Autodesk Inventor part; units mm, degrees
ref_plane "YZ Plane" through (0, 0, 0) normal (1, 0, 0) x (0, 1, 0)
ref_plane "XZ Plane" through (0, 0, 0) normal (0, 1, 0) x (-1, 0, 0)
ref_plane "XY Plane" through (0, 0, 0) normal (0, 0, 1) x (1, 0, 0)
sketch "Sketch1" plane through (0, 0, 0) normal (0, 0, 1) x (1, 0, 0)
  circle A0 centre (0, 0) radius 3.4925
  dimension "d0" = 6.985
extrude "Extrusion1" add sketch "Sketch1" along normal blind 2.54
sketch "Sketch2" plane through (0, 0, 2.54) normal (0, 0, 1) x (1, 0, 0)
  circle A0 centre (0, 0) radius 3.4925
  circle A1 centre (0, 0) radius 1.905
  dimension "d3" = 3.81
extrude "Extrusion2" add sketch "Sketch2" along normal blind 8.255 contours A1
sketch "Sketch3" plane through (0, 0, 0) normal (0, 0, -1) x (-1, 0, 0)
  circle A0 centre (0, 0) radius 3.4925
  line L0 (1.4665, 0) -> (0.7332, -1.27)
  line L1 (0.7332, -1.27) -> (-0.7332, -1.27)
  line L2 (-0.7332, -1.27) -> (-1.4665, 0)
  line L3 (-1.4665, 0) -> (-0.7332, 1.27)
  line L4 (-0.7332, 1.27) -> (0.7332, 1.27)
  line L5 (0.7332, 1.27) -> (1.4665, 0)
  dimension "d6" = 2.54
extrude "Extrusion3" cut sketch "Sketch3" against normal blind 2.54 contours L0 L1 L2 L3 L4 L5
thread "Thread1"
fillet "Fillet1" radius 0.254 3 edges at (-3.4925, 0, 0) (-3.4925, 0, 2.54) (-1.905, 0, 10.795)
properties part number "20mm T-Nut Fastener 1764"
Could you check a few things on this model? Use its own coordinates, in mm. A direction names the side the tool comes from. Round coordinates to 2 decimals unless told otherwise and drop trailing zeros. Order: outer loops, then holes, each group sorted by start corner. A loop starts at its lowest first (then second) coordinate and runs counter-clockwise, first axis right, second up.
(1) Imagine slicing it at A-A (z = 1.75). Write out the boundary of the cut face in (x, y) (1 decimal), plus the area to 3 significant figures.
Response values:
outline: circle Ø7 at (0, 0); hole (-1.5, 0) - (-0.7, -1.3) - (0.7, -1.3) - (1.5, 0) - (0.7, 1.3) - (-0.7, 1.3) - close
area: 32.7 mm2
(2) I'm going to push flat-ended pins straight in: pin 1 (1.3 mm diameter, centred on x = -0.5, y = -0.5, fed in from -Z); pin 2 (1 mm diameter, centred on y = 2, z = 7, fed in from -X); pin 3 (1.5 mm diameter, centred on y = 2, z = 9, fed in from -X); pin 4 (2 mm diameter, centred on x = -2.5, y = -2.5, fed in from +Z). Where does each tip first touch, or does it pass through?
Response values:
pin 1: stops at z = 0
pin 2: stops at x = -1.17
pin 3: stops at x = -1.44
pin 4: stops at z = 2.54
(3) Imagine slicing it at C-C (z = 4). Write out the boundary of the cut face in (x, y) (3 decimals).
Response values:
outline: circle Ø3.81 at (0, 0)
(4) Which directions (+Z, -Z, +X, -X, +Y, -Y) give clear straight access to the entire face, cutting with the end or side of a thin tool? Please do faces 1 (the flat face through (0, -2.1, 2.54)), 2 (the cylindrical face through (-0.455, -3.463, 1.256)), 3 (the flat face through (1.105, 0.626, 1.252)).
Response values:
face 1: +Z
face 2: +Z, -Z
face 3: -Z
(5) Please list where these lines run through material, in increasing order: line 1 along Z through (x, y) = (2, 1); line 2 along Z through (x, y) = (0.25, 0.25) (3 decimals); line 3 along X through (y, z) = (0.75, 0.5).
Response values:
line 1: z = 0 to 2.54
line 2: z = 2.54 to 10.795
line 3: x = -3.41 to -1.03, 1.03 to 3.41
(6) If we mould it in two halves opening along Y, with no side actions, what happens to faces 4 (the cylindrical face through (-0.41, 1.86, 6.48)), 5 (the flat face through (1.4, -0.7, 0)), 6 (the flat face through (0, 0, 2.54)), 7 (the flat face through (-1.095, 0.644, 1.252))? For each: released by +Y, released by -Y, zero draft, split by the parting line, or undercut.
Response values:
face 4: split by the parting line
face 5: zero draft
face 6: undercut
face 7: undercut
